Print and shaded views of the part. All mm, measured from the part's lowest x, y and z. Round coordinates to 2 decimals unless told otherwise and drop trailing zeros. Loops run counter-clockwise (first coordinate to the right, second up) from the corner with the lowest first, then second, coordinate; pieces in that order, holes last. Notation, with made-up numbers: (-19, -7) - (21, -7) arc R34 ccw to (21, 27) - close; hole circle Ø9 at (57.5, 9). An arc over 180 degrees is marked (long way). Use one line per item in the form item = value.
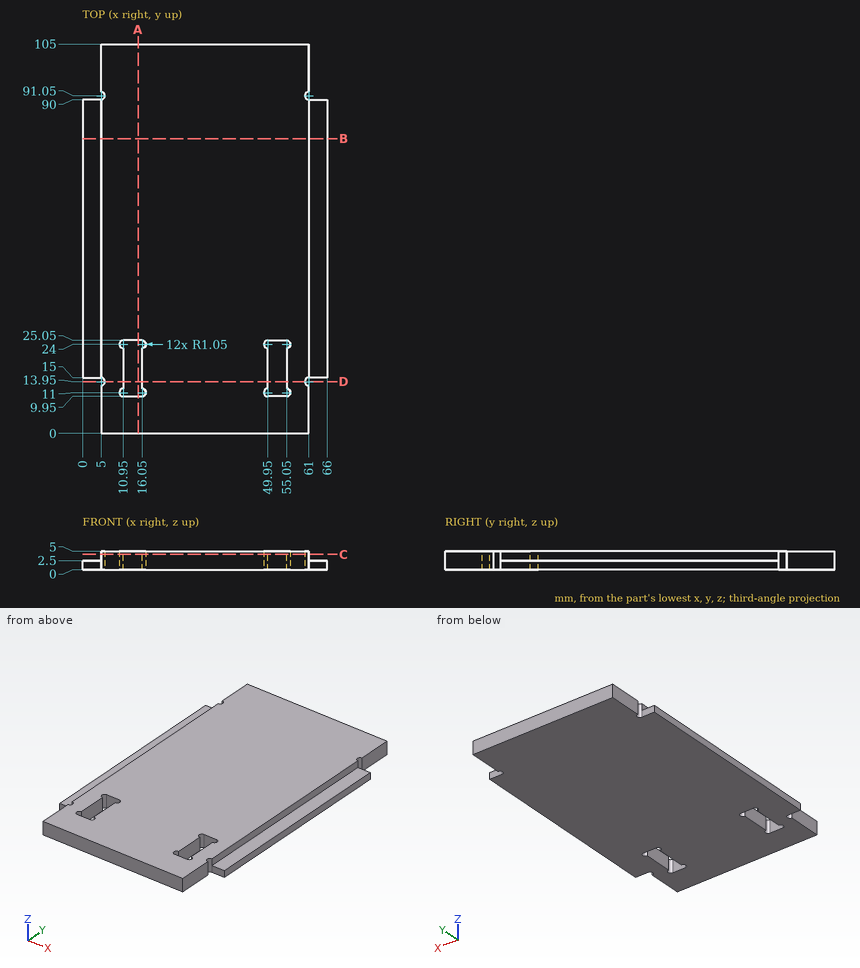
1) Slice it at C-C (z = 4.2). Write the cut outline in (x, y).
Report:
outline = (5, 0) - (61, 0) - (61, 12.9) arc R1.05 cw to (61, 15) - (61, 90) arc R1.05 cw to (61, 92.1) - (61, 105) - (5, 105) - (5, 92.1) arc R1.05 cw to (5, 90) - (5, 15) arc R1.05 cw to (5, 12.9) - close; hole (10.95, 9.95) - (16.05, 9.95) arc R1.05 ccw to (16.05, 12.05) - (16.05, 22.95) arc R1.05 ccw to (16.05, 25.05) - (10.95, 25.05) arc R1.05 ccw to (10.95, 22.95) - (10.95, 12.05) arc R1.05 ccw to start; hole (49.95, 9.95) - (55.05, 9.95) arc R1.05 ccw to (55.05, 12.05) - (55.05, 22.95) arc R1.05 ccw to (55.05, 25.05) - (49.95, 25.05) arc R1.05 ccw to (49.95, 22.95) - (49.95, 12.05) arc R1.05 ccw to start
2) Slice it at A-A (x = 15). Write the cut outline in (y, z), plus the area to 4 significant figures.
Report:
outline = (0, 0) - (9.95, 0) - (9.95, 5) - (0, 5) - close; (25.05, 0) - (105, 0) - (105, 5) - (25.05, 5) - close
area = 449.5 mm^2
3) Flat gauge pins, fed straight in: pin 1 (5.5 mm diameter, centred on x = 3, y = 64.5, fed in from +Z); pin 2 (1.2 mm diameter, centred on y = 71, z = 4, fed in from -X); pin 3 (3 mm diameter, centred on x = 63, z = 1.5, fed in from +Y); pin 4 (0.8 mm diameter, centred on x = 2, z = 1, fed in from -Y). Where does each tip first touch, or does it go through?
Report:
pin_1 = 5
pin_2 = 5
pin_3 = 90
pin_4 = 15
4) Slice it at D-D (y = 13.95). Write the cut outline in (x, z).
Report:
outline = (6.05, 0) - (10.95, 0) - (10.95, 5) - (6.05, 5) - close; (16.05, 0) - (49.95, 0) - (49.95, 5) - (16.05, 5) - close; (55.05, 0) - (59.95, 0) - (59.95, 5) - (55.05, 5) - close
5) Drill centre lines: probe 1 along X at (y, z) = (17, 3.7); probe 2 along Y at (x, z) = (50.5, 2); probe 3 along X at (y, z) = (5, 2.1). Where is each one in solid material? Low to high.
Report:
probe_1 = 5 to 10.95, 16.05 to 49.95, 55.05 to 61
probe_2 = 0 to 9.95, 25.05 to 105
probe_3 = 5 to 61
6) Slice it at B-B (y = 79.5). Write the cut outline in (x, z).
Report:
outline = (0, 0) - (66, 0) - (66, 2.5) - (61, 2.5) - (61, 5) - (5, 5) - (5, 2.5) - (0, 2.5) - close
